Can you work these out from the model? Positions are in its coordinate system, mm. Face numbers are marked on the shaded views. A direction names the side the tool comes from. Coordinates: 2 decimals unless noted, no trailing zeros. Loops run counter-clockwise (first coordinate to the right, second up) from the corner with the lowest first, then second, coordinate; pieces in that order, holes last. Notation, with made-up numbers: (-2.75, 67) -> (46.25, 67) arc R23 ccw to (46.25, 75) -> close; hole circle Ø2 at (63, 36). An arc over 180 degrees is marked (long way). Use one line per item in the form item = value. Start each with the question number.
(1) Imagine slicing it at D-D (x = -3). List the corners of the cut face in (y, z) for me.
(2) On a 3-axis mill with a long thin cutter (end or side, diameter ignored), from which of +Z, -Z, +X, -X, +Y, -Y can I reach the whole of each face in a straight line? I mean the marked faces 1, 2, 3, 4 and 5. Say none if no direction works.
(3) I need wall thicknesses on line 1 (X direction, y = 62.5, z = 65.5); line 2 (X direction, y = 7, z = 70.5); line 3 (X direction, y = 44, z = 103). Which ranges of each line are inside material? Lowest first, please. Write a range as [from, to].
(4) Imagine slicing it at A-A (z = 57.5). List the corners of the cut face in (x, y) for me, plus the area to 3 significant figures.
(5) Imagine slicing it at B-B (y = 9.5). List the corners of the cut face in (x, z) for me, plus the area to 3 significant figures.
(6) Imagine slicing it at C-C (z = 140). List the corners of the cut face in (x, y) for me.
(7) I'm going to push flat-ended pins straight in: pin 1 (19 mm diameter, centred on y = -2.5, z = 38, fed in from +X); pin 2 (12 mm diameter, centred on y = 1.5, z = 70, fed in from +X); pin 3 (0.9 mm diameter, centred on x = -2, z = 149, fed in from +Y). Where does each tip first touch, or does it pass through?
(8) Thinking about a two-plate mould opening in X: for the marked faces 6, 7, 8 and 9, which applies, released by +X, released by -X, zero draft, split by the parting line, or undercut?
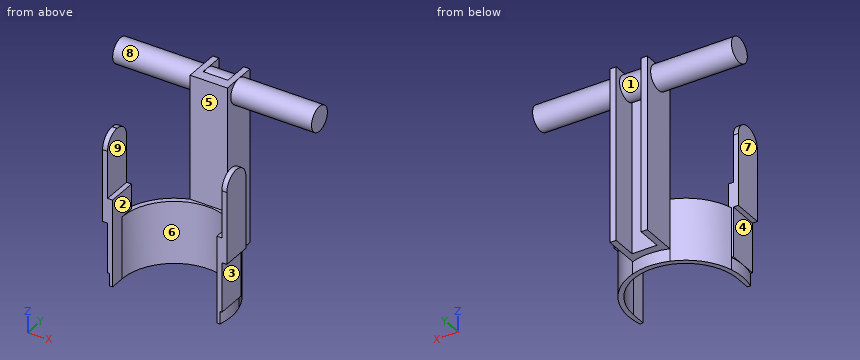
```python
from build123d import *

# Parameters (mm, degrees)
EXTRUDE_1_DEPTH     = 50
SKETCH_3_W          = 4
SKETCH_3_H          = 24
EXTRUDE_2_DEPTH     = 70
SKETCH_5_R          = 80
SKETCH_5_R_2        = 46
CUT_EXTRUDE_2_DEPTH = 10
EXTRUDE_4_DEPTH     = 140
SKETCH_10_R         = 10
EXTRUDE_5_DEPTH     = 80
SKETCH_12_W         = 4
SKETCH_12_H         = 70
EXTRUDE_6_DEPTH     = 24
CUT_EXTRUDE_3_DEPTH = 131


with BuildPart() as part:
    # 草图2 → 凸台-拉伸1 (new body)
    with BuildSketch(Plane.XY):
        with BuildLine():
            Line((-46, 0), (-42, 0))
            ThreePointArc((-42, 0), (0, 42), (42, 0))
            Line((42, 0), (46, 0))
            ThreePointArc((46, 0), (37.456641601, 26.702059846), (15, 43.48562981))
            Line((15, 43.48562981), (15, 72))
            Line((15, 72), (10, 72))
            Line((10, 72), (10, 52))
            Line((10, 52), (-10, 52))
            Line((-10, 52), (-10, 72))
            Line((-10, 72), (-15, 72))
            Line((-15, 72), (-15, 43.48562981))
            ThreePointArc((-15, 43.48562981), (-37.456641601, 26.702059846), (-46, 0))
        make_face()
    extrude(amount=EXTRUDE_1_DEPTH)

    # 草图3 → 凸台-拉伸2 (add)
    with BuildSketch(Plane(origin=(0, 0, 0), x_dir=(-1, 0, 0), z_dir=(0, 0, -1))):
        with Locations((-44, 0)):
            Rectangle(SKETCH_3_W, SKETCH_3_H)
        with Locations((44, 0)):
            Rectangle(SKETCH_3_W, SKETCH_3_H)
    extrude(amount=-EXTRUDE_2_DEPTH)

    # 草图5 → 切除-拉伸2 (cut)
    with BuildSketch(Plane(origin=(0, 0, 0), x_dir=(-1, 0, 0), z_dir=(0, 0, -1))):
        Circle(SKETCH_5_R)
        Circle(SKETCH_5_R_2, mode=Mode.SUBTRACT)
    extrude(amount=-CUT_EXTRUDE_2_DEPTH, mode=Mode.SUBTRACT)

    # 草图9 → 凸台-拉伸4 (add)
    with BuildSketch(Plane(origin=(0, 0, 10), x_dir=(-1, 0, 0), z_dir=(0, 0, -1))):
        Polygon((-15, 72), (-15, 43.48562981), (15, 43.48562981), (15, 72), (10, 72), (10, 52), (-10, 52), (-10, 72), align=None)
    extrude(amount=-EXTRUDE_4_DEPTH)

    # 草图10 → 凸台-拉伸5 (add, symmetric)
    with BuildSketch(Plane(origin=(0, 0, 0), x_dir=(0, 0, -1), z_dir=(1, 0, 0))):
        with Locations((-140, 57.742814905)):
            Circle(SKETCH_10_R)
    extrude(amount=EXTRUDE_5_DEPTH, both=True)

    # 草图12 → 凸台-拉伸6 (add)
    with BuildSketch(Plane.XZ.offset(12)):
        with Locations((-48, 84.999732959)):
            Rectangle(SKETCH_12_W, SKETCH_12_H)
        with Locations((48, 85)):
            Rectangle(SKETCH_12_W, SKETCH_12_H)
    extrude(amount=-EXTRUDE_6_DEPTH)

    # 草图13 → 切除-拉伸3 (cut, through all)
    with BuildSketch(Plane.ZY.offset(50)):
        with BuildLine():
            Line((108, 12), (128.196913472, 12))
            Line((128.196913472, 12), (128.196913472, -12))
            Line((128.196913472, -12), (108, -12))
            ThreePointArc((108, -12), (120, 0), (108, 12))
        make_face()
    extrude(amount=-CUT_EXTRUDE_3_DEPTH, mode=Mode.SUBTRACT)


solid = part.part
```
Worked out:
q1.outline = (41.89, 0) -> (45.9, 0) -> (45.9, 10) -> (52, 10) -> (52, 131.81) arc R10 ccw (long way) to (52, 148.19) -> (52, 150) -> (43.49, 150) -> (43.49, 50) -> (41.89, 50) -> close
q2.face_1 = none
q2.face_2 = +Z, -Y
q2.face_3 = -Z, +X, +Y, -Y
q2.face_4 = -Z, -X, +Y, -Y
q2.face_5 = +Z, +X, -X, -Y
q3.line_1 = [-15, -10], [10, 15]
q3.line_2 = [-50, -46], [46, 50]
q3.line_3 = [-15, 15]
q4.outline = (-50, -12) -> (-42, -12) -> (-42, 12) -> (-50, 12) -> close; (-15, 43.49) -> (15, 43.49) -> (15, 72) -> (10, 72) -> (10, 52) -> (-10, 52) -> (-10, 72) -> (-15, 72) -> close; (42, -12) -> (50, -12) -> (50, 12) -> (42, 12) -> close
q4.area = 839 mm2
q5.outline = (-50, 50) -> (-46, 50) -> (-46, 10) -> (-45.01, 10) -> (-45.01, 0) -> (-40.91, 0) -> (-40.91, 50) -> (-42, 50) -> (-42, 70) -> (-46, 70) -> (-46, 115.33) -> (-50, 115.33) -> close; (40.91, 0) -> (45.01, 0) -> (45.01, 10) -> (46, 10) -> (46, 50) -> (50, 50) -> (50, 115.33) -> (46, 115.33) -> (46, 70) -> (42, 70) -> (42, 50) -> (40.91, 50) -> close
q5.area = 1,170 mm2
q6.outline = (-80, 47.74) -> (-15, 47.74) -> (-15, 43.49) -> (15, 43.49) -> (15, 47.74) -> (80, 47.74) -> (80, 67.74) -> (15, 67.74) -> (15, 72) -> (10, 72) -> (10, 67.74) -> (-10, 67.74) -> (-10, 72) -> (-15, 72) -> (-15, 67.74) -> (-80, 67.74) -> close
q7.pin_1 = 46
q7.pin_2 = 50
q7.pin_3 = 62.93
q8.face_6 = undercut
q8.face_7 = released by -X
q8.face_8 = zero draft
q8.face_9 = undercut
